Read the model definition and answer for the solid it produces. Units are mm, in the model's axes. Round coordinates to 2 decimals unless told otherwise and drop trailing zeros. Write each loop counter-clockwise with the first axis right and the second up, starting at its lowest first coordinate (ties: lowest second). Pieces come first, ordered by that corner, then holes.
from build123d import *

# Parameters (mm, degrees)
F0_W     = 1041.4
F0_H     = 241.3
F0_R     = 79.375
F0_R_2   = 70.485
F1_DEPTH = 19.05
F2_R     = 12.7


with BuildPart() as f1:
    # F0 (on Front) → F1 (new body)
    with BuildSketch(Plane.XZ):
        with Locations((17.794014, -118.442795)):
            Rectangle(F0_W, F0_H)
        with Locations((-388.605986, -118.442795)):
            Circle(F0_R, mode=Mode.SUBTRACT)
        with Locations((-185.405986, -118.442795)):
            Circle(F0_R_2, mode=Mode.SUBTRACT)
        with Locations((17.794014, -118.442795)):
            Circle(F0_R_2, mode=Mode.SUBTRACT)
        with Locations((220.994014, -118.442795)):
            Circle(F0_R_2, mode=Mode.SUBTRACT)
        with Locations((424.194014, -118.442795)):
            Circle(F0_R_2, mode=Mode.SUBTRACT)
    extrude(amount=F1_DEPTH)

    # F2
    f2_edges = [f1.edges().sort_by_distance(p)[0] for p in [
        (17.794014, -19.05, 2.207205),
        (-502.905986, -19.05, -118.442795),
        (17.794014, -19.05, -239.092795),
        (538.494014, -19.05, -118.442795),
    ]]
    fillet(f2_edges, radius=F2_R)


solid = f1.part
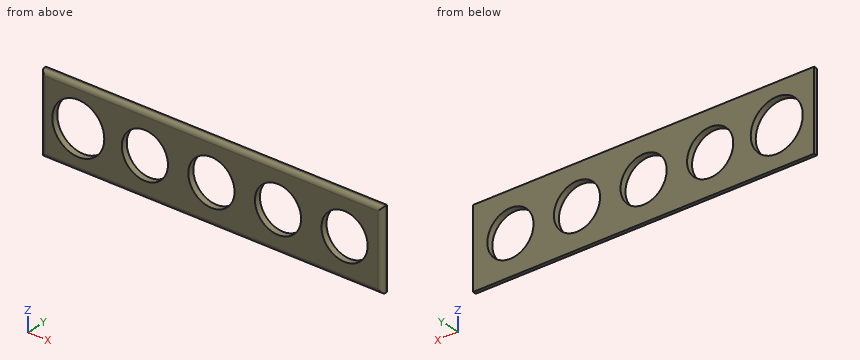
Q1. Section C-C (y = -14.5) is taken. Determine the outline of the cut face in (x, z) (3 decimals).
Verdict:
outline: (-499.946, -236.133) - (535.534, -236.133) - (535.534, -0.753) - (-499.946, -0.753) - close; hole circle Ø158.75 at (-388.606, -118.443); hole circle Ø140.97 at (-185.406, -118.443); hole circle Ø140.97 at (17.794, -118.443); hole circle Ø140.97 at (220.994, -118.443); hole circle Ø140.97 at (424.194, -118.443)
Q2. Section B-B (z = -134) is taken. Determine the outline of the cut face in (x, y).
Verdict:
outline: (-502.91, -6.35) arc R12.7 ccw to (-490.21, -19.05) - (-466.44, -19.05) - (-466.44, 0) - (-502.91, 0) - close; (-310.77, -19.05) - (-254.15, -19.05) - (-254.15, 0) - (-310.77, 0) - close; (-116.66, -19.05) - (-50.95, -19.05) - (-50.95, 0) - (-116.66, 0) - close; (86.54, -19.05) - (152.25, -19.05) - (152.25, 0) - (86.54, 0) - close; (289.74, -19.05) - (355.45, -19.05) - (355.45, 0) - (289.74, 0) - close; (492.94, -19.05) - (525.79, -19.05) arc R12.7 ccw to (538.49, -6.35) - (538.49, 0) - (492.94, 0) - close
Q3. Flat-ended cylindrical pins translate along their axes: pin 1 Ø1.5 at (y, z) = (-11.5, -202.5) entering from -X; pin 2 Ø1.5 at (x, y) = (284.5, -7.5) entering from +Z; pin 3 Ø8 at (y, z) = (-10.5, -166.5) entering from +X; pin 4 Ø5 at (y, z) = (-15, -23) entering from +X. Find the tip coordinate at first contact, or state that the pin passes through.
Verdict:
pin 1: stops at x = -502.12
pin 2: stops at z = 2.2
pin 3: stops at x = 538.49
pin 4: stops at x = 536.91
Q4. Section A-A (x = 190) is taken. Determine the outline of the cut face in (y, z).
Verdict:
outline: (-19.05, -226.39) arc R12.7 ccw to (-6.35, -239.09) - (0, -239.09) - (0, -181.75) - (-19.05, -181.75) - close; (-19.05, -55.14) - (0, -55.14) - (0, 2.21) - (-6.35, 2.21) arc R12.7 ccw to (-19.05, -10.49) - close
Q5. Straight lines are drawn through the part: probe 1 along X at (y, z) = (-8, -161.5); probe 2 along X at (y, z) = (-1.25, -174); probe 3 along Z at (x, y) = (26, -16). For each, find the intervals that lie inside material, in ascending order.
Verdict:
probe 1: x = -502.8 to -455.29, -321.92 to -241.21, -129.6 to -38.01, 73.6 to 165.19, 276.8 to 368.39, 480 to 538.39
probe 2: x = -502.91 to -445.3, -331.92 to -228.78, -142.03 to -25.58, 61.17 to 177.62, 264.37 to 380.82, 467.57 to 538.49
probe 3: z = -234.65 to -188.45, -48.44 to -2.24
Q6. Section D-D (x = -16) is taken. Determine the outline of the cut face in (y, z).
Verdict:
outline: (-19.05, -226.39) arc R12.7 ccw to (-6.35, -239.09) - (0, -239.09) - (0, -180.3) - (-19.05, -180.3) - close; (-19.05, -56.59) - (0, -56.59) - (0, 2.21) - (-6.35, 2.21) arc R12.7 ccw to (-19.05, -10.49) - close
